Can you work these out from the model? Positions are in its coordinate system, mm. A direction names the side the tool comes from. Give positions to 0.01 mm unless a question says otherwise; leave off trailing zeros. One line per item, written item: value.
from build123d import *

# Parameters (mm, degrees)
F1_DEPTH = 53
F2_R     = 0.1
F3_R     = 1.40385
F4_DEPTH = 10


with BuildPart() as f1:
    # F0 (on Top) → F1 (new body)
    with BuildSketch(Plane.XY):
        Polygon((0.5, 5), (0, 5), (-0.5, 5), (-0.8, 2.3), (-1.06066, 2.192031), (-3.181981, 3.889087), (-3.535534, 3.535534), (-3.889087, 3.181981), (-2.192031, 1.06066), (-2.3, 0.8), (-5, 0.5), (-5, 0), (-5, -0.5), (-2.3, -0.8), (-2.192031, -1.06066), (-3.889087, -3.181981), (-3.535534, -3.535534), (-3.181981, -3.889087), (-1.06066, -2.192031), (-0.8, -2.3), (-0.5, -5), (0, -5), (0.5, -5), (0.8, -2.3), (1.06066, -2.192031), (3.181981, -3.889087), (3.535534, -3.535534), (3.889087, -3.181981), (2.192031, -1.06066), (2.3, -0.8), (5, -0.5), (5, 0), (5, 0.5), (2.3, 0.8), (2.192031, 1.06066), (3.889087, 3.181981), (3.535534, 3.535534), (3.181981, 3.889087), (1.06066, 2.192031), (0.8, 2.3), align=None)
    extrude(amount=F1_DEPTH)

    # F2
    f2_edges = [f1.edges().sort_by_distance(p)[0] for p in [
        (3.889087, 3.181981, 26.5),
        (3.181981, 3.889087, 26.5),
        (5, 0.5, 26.5),
        (5, -0.5, 26.5),
        (3.889087, -3.181981, 26.5),
        (3.181981, -3.889087, 26.5),
        (-3.889087, -3.181981, 26.5),
        (-3.181981, -3.889087, 26.5),
        (-0.5, -5, 26.5),
        (0.5, -5, 26.5),
        (-5, -0.5, 26.5),
        (-5, 0.5, 26.5),
        (-3.889087, 3.181981, 26.5),
        (-3.181981, 3.889087, 26.5),
        (-0.5, 5, 26.5),
        (0.5, 5, 26.5),
    ]]
    fillet(f2_edges, radius=F2_R)


with BuildPart() as f4:
    # F3 (on face) → F4 (new body)
    with BuildSketch(Plane(origin=(0, 0, 0), x_dir=(1, 0, 0), z_dir=(0, 0, -1))):
        Circle(F3_R)
    extrude(amount=F4_DEPTH)


solid = f1.part
1) I need wall thicknesses on L1, parallel to Y at x = -2.5, z = 6.5; L2, parallel to X at y = 3, z = 9.5; L3, parallel to Y at x = 3.5, z = 19.5. Which ranges of each line are inside material? Lowest first, please.
Answer list:
L1: y = -3.34 to -1.45, -0.78 to 0.78, 1.45 to 3.34
L2: x = -3.74 to -2.07, -0.72 to 0.72, 2.07 to 3.74
L3: y = -3.57 to -2.7, -0.67 to 0.67, 2.7 to 3.57
2) Will this pin go through, and if not, where does the flat tip stop? pin 1 (2 mm diameter, centred on y = 3.5, z = 28, fed in from -X).
Answer list:
pin 1: stops at x = -3.86
3) We'd pull the mould along Y, two halves only. Please class faces 1 (the face through (0.657, 3.587, 26.129)), 2 (the face through (-0.657, -3.587, 26.129)), 3 (the face through (-3.587, 0.657, 26.129)): released by +Y, released by -Y, zero draft, split by the parting line, or undercut.
Answer list:
face 1: released by +Y
face 2: released by -Y
face 3: undercut
4) For faces 4 (the face through (-2.07, 3, 26.13)), 5 (the face through (0, 0, 0)), 6 (the face through (3, 2.07, 26.13)), 7 (the face through (2.07, -3, 26.13)), 8 (the face through (-3, -2.07, 26.13)), which set-ups out of +Z, -Z, +X, -X, +Y, -Y let a thin tool reach every point of the face, with its end or its side?
Answer list:
face 4: +Z, -Z, +Y
face 5: -Z, +X, -X, +Y, -Y
face 6: +Z, -Z, +X
face 7: +Z, -Z, -Y
face 8: +Z, -Z, -X
